Could you check a few things on this drawing? It's one solid part, dimensions in mm from its lowest x, y, z. A direction names the side the tool comes from. Give positions to 0.01 mm unless a question says otherwise; leave off trailing zeros. Order: outer loops, then holes, each group sorted by start corner. A loop starts at its lowest first (then second) coordinate and runs counter-clockwise, first axis right, second up. Notation, with made-up numbers: (48.25, -2.75) -> (57.25, -2.75) arc R28 cw to (57.25, 29.25) -> close; hole circle Ø1 at (-12, 42). An arc over 180 degrees is marked (long way). Use one line per item in the form item = value. Start each with the question number.
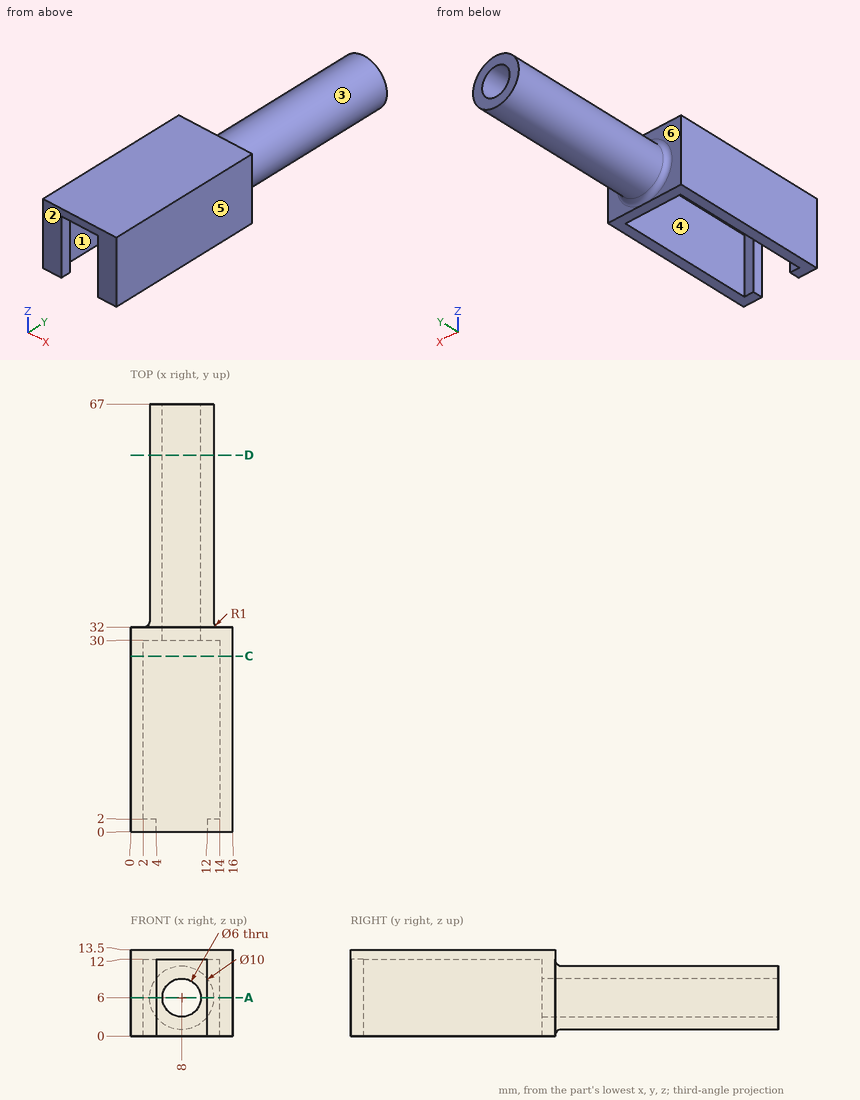
(1) Imagine slicing it at D-D (y = 59). Write out the boundary of the cut face in (x, z).
(2) Which directions (+Z, -Z, +X, -X, +Y, -Y) give clear straight access to the entire face, cutting with the end or side of a thin tool? Please do the marked faces 4, 5 and 6.
(3) I'm going to push flat-ended pins straight in: pin 1 Ø0.6 at (x, z) = (13.5, 6) entering from +Y; pin 2 Ø3.5 at (x, z) = (7, 8) entering from -Y; pin 3 Ø4 at (x, z) = (2, 11.5) entering from +Y. Where does each tip first touch, or does it pass through?
(4) Imagine slicing it at A-A (z = 6). Write out the boundary of the cut face in (x, y), plus the area to 3 significant figures.
(5) We'd pull the mould along Y, two halves only. Please class the marked faces 1, 2 and 3: pulls with the +Y half, pulls with the -Y half, needs draft (parallel to the pull), parting line crosses it, or undercut.
(6) Imagine slicing it at C-C (y = 27.5). Write out the boundary of the cut face in (x, z), plus the area to 3 significant figures.
(7) Please list where these lines run through material, in increasing order: probe 1 along X at (y, z) = (12.5, 3.25); probe 2 along X at (y, z) = (41, 6); probe 3 along Y at (x, z) = (3.5, 1.25).
Calculated:
q1.outline = circle Ø10 at (8, 6); hole circle Ø6 at (8, 6)
q2.face_4 = -Z
q2.face_5 = +Z, -Z, +X, +Y, -Y
q2.face_6 = +Y
q3.pin_1 = 32.4
q3.pin_2 = 30
q3.pin_3 = 32
q4.outline = (0, 0) -> (4, 0) -> (4, 2) -> (2, 2) -> (2, 30) -> (5, 30) -> (5, 67) -> (3, 67) -> (3, 33) arc R1 cw to (2, 32) -> (0, 32) -> close; (11, 30) -> (14, 30) -> (14, 2) -> (12, 2) -> (12, 0) -> (16, 0) -> (16, 32) -> (14, 32) arc R1 cw to (13, 33) -> (13, 67) -> (11, 67) -> close
q4.area = 288 mm2
q5.face_1 = undercut
q5.face_2 = pulls with the -Y half
q5.face_3 = needs draft
q6.outline = (0, 0) -> (2, 0) -> (2, 12) -> (14, 12) -> (14, 0) -> (16, 0) -> (16, 13.5) -> (0, 13.5) -> close
q6.area = 72.0 mm2
q7.probe_1 = 0 to 2, 14 to 16
q7.probe_2 = 3 to 5, 11 to 13
q7.probe_3 = 0 to 2, 30 to 32
